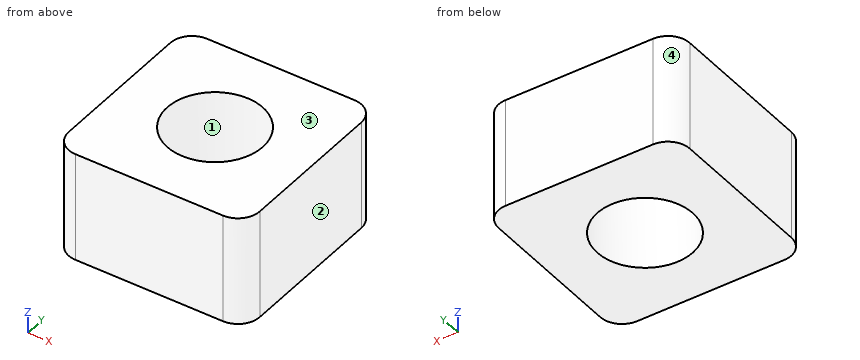
Solid Edge part; units mm, degrees
sketch "Sketch1" plane through (0, 0, 0) normal (0, 0, 1) x (1, 0, 0)
  line L0 (-35, -35) -> (35, -35)
  line L1 (35, -35) -> (35, 35)
  line L2 (35, 35) -> (-35, 35)
  line L3 (-35, 35) -> (-35, -35)
extrude "ExtrudedProtrusion_1" add sketch "Sketch1" along normal blind 40
fillet "Round_1" radius 8 4 edges at (35, -35, 20) (35, 35, 20) (-35, -35, 20) (-35, 35, 20)
sketch "Sketch2" plane through (0, 0, 0) normal (0, 0, 1) x (1, 0, 0)
  circle A0 centre (0, 0) radius 17.5
extrude "ExtrudedCutout_1" cut sketch "Sketch2" along normal blind 118.7913
Read the model definition and answer for the solid it produces. Units are mm, in the model's axes. Face numbers are marked on the shaded views. Give positions to 0.01 mm unless a question says otherwise; leave off trailing zeros. Write each loop counter-clockwise with the first axis right and the second up, starting at its lowest first coordinate (ties: lowest second). Pieces come first, ordered by that corner, then holes. Notation, with made-up numbers: M -37.75,-23.5 L -22.75,-23.5 A24 cw -22.75,-3.5 Z; hole C 84.25,25.5 d1. An arc over 180 degrees is marked long. One line per item, written item: value. Start each with the question number.
(1) Find section C-C (z = 3.5). Determine the outline of the cut face in (x, y).
(2) Find the intervals of material crossed by line 1 (Y direction, x = 0, z = 22.5); line 2 (X direction, y = 8, z = 17), in increasing order.
(3) Determine the mould class of the marked faces 1, 2, 3 and 4 for opening direction X: pulls with the +X half, pulls with the -X half, needs draft (parallel to the pull), parting line crosses it, or undercut.
(4) Find section A-A (y = 0). Determine the outline of the cut face in (x, z), plus the area to 3 significant figures.
Results below:
1. outline: M -35,-27 A8 ccw -27,-35 L 27,-35 A8 ccw 35,-27 L 35,27 A8 ccw 27,35 L -27,35 A8 ccw -35,27 Z; hole C 0,0 d35
2. line 1: y = -35 to -17.5, 17.5 to 35
2. line 2: x = -35 to -15.56, 15.56 to 35
3. face 1: undercut
3. face 2: pulls with the +X half
3. face 3: needs draft
3. face 4: pulls with the -X half
4. outline: M -35,0 L -17.5,0 L -17.5,40 L -35,40 Z; M 17.5,0 L 35,0 L 35,40 L 17.5,40 Z
4. area: 1,400 mm^2
